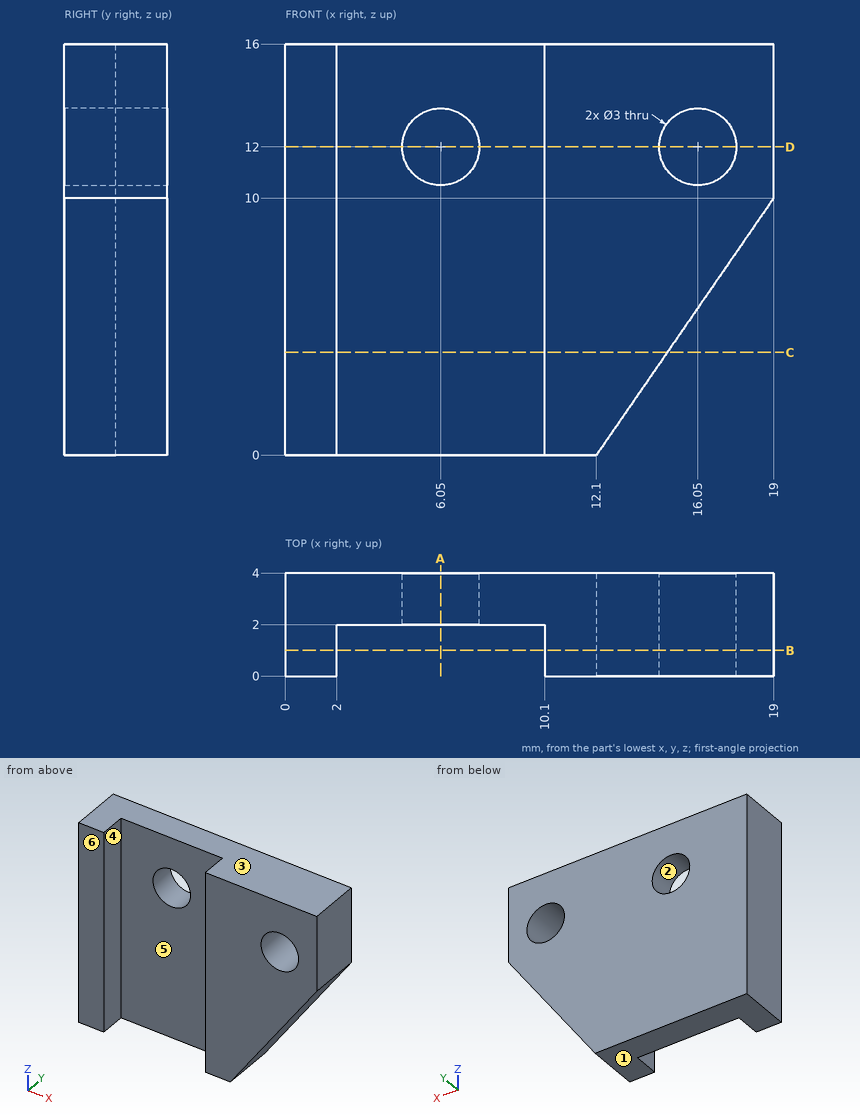
Print and shaded views of the part. All mm, measured from the part's lowest x, y and z. A direction names the side the tool comes from. Give positions to 0.01 mm unless a question says otherwise; leave off trailing zeros. Loops run counter-clockwise (first coordinate to the right, second up) from the corner with the lowest first, then second, coordinate; pieces in that order, holes last.
1) Flat gauge pins, fed straight in: pin 1 Ø1.6 at (y, z) = (1.5, 4.5) entering from +X; pin 2 Ø1.8 at (x, z) = (16.05, 12) entering from +Y; pin 3 Ø4 at (x, z) = (7.5, 9.5) entering from -Y. Where does each tip first touch, or does it go through?
2) Wall check: line 1 (X direction, y = 0.8, z = 12); line 2 (X direction, y = 3.5, z = 12); line 3 (Y direction, x = 6, z = 6.5). Give the ranges that are in metal, low to high.
3) Pull direction Z, two halves, no side cores. Call the marked faces 1, 2, 3 and 4: +Z half, -Z half, draft (parallel to the pull), parting line (faces both ways), or undercut.
4) Saw through at A-A (x = 6.05). Write the cut outline in (y, z).
5) Saw through at D-D (z = 12). Write the cut outline in (x, y), plus the area to 3 significant figures.
6) Saw through at C-C (z = 4). Write the cut outline in (x, y), plus the area to 3 significant figures.
7) Tool access for the marked faces 5 and 6: list every direction of +Z, -Z, +X, -X, +Y, -Y with a clear straight run to the whole face (end or side of a thin tool).
8) Saw through at B-B (y = 1). Write the cut outline in (x, z), plus the area to 3 significant figures.
Answer block:
1. pin 1: stops at x = 15.76
1. pin 2: passes through
1. pin 3: stops at y = 2
2. line 1: x = 0 to 2, 10.1 to 14.55, 17.55 to 19
2. line 2: x = 0 to 4.55, 7.55 to 14.55, 17.55 to 19
2. line 3: y = 2 to 4
3. face 1: -Z half
3. face 2: undercut
3. face 3: +Z half
3. face 4: draft
4. outline: (2, 0) - (4, 0) - (4, 10.5) - (2, 10.5) - close; (2, 13.5) - (4, 13.5) - (4, 16) - (2, 16) - close
5. outline: (0, 0) - (2, 0) - (2, 2) - (4.55, 2) - (4.55, 4) - (0, 4) - close; (7.55, 2) - (10.1, 2) - (10.1, 0) - (14.55, 0) - (14.55, 4) - (7.55, 4) - close; (17.55, 0) - (19, 0) - (19, 4) - (17.55, 4) - close
5. area: 41.8 mm2
6. outline: (0, 0) - (2, 0) - (2, 2) - (10.1, 2) - (10.1, 0) - (14.86, 0) - (14.86, 4) - (0, 4) - close
6. area: 43.2 mm2
7. face 5: +Z, -Z, -Y
7. face 6: +Z, -Z, +X, -X, -Y
8. outline: (0, 0) - (2, 0) - (2, 16) - (0, 16) - close; (10.1, 0) - (12.1, 0) - (19, 10) - (19, 16) - (10.1, 16) - close; hole circle Ø3 at (16.05, 12)
8. area: 133 mm2
